Source: CAD feature listing. Evaluate the final solid. Frame: model axes, mm. Face numbers are marked on the shaded views. Coordinates: 2 decimals unless noted, no trailing zeros. Write each loop counter-clockwise with the first axis right and the second up, starting at its lowest first coordinate (ties: lowest second). Pieces come first, ordered by that corner, then holes. Notation, with made-up numbers: M -38,31 L 2,31 A28 cw 2,68 Z; hole C -25.75,38 d8. An arc over 180 degrees is marked long. One line per item, written item: value. Start each with the question number.
Item 1: Pin query (flat end, axial travel): P1, Ø0.7, axis at y = 0.5, z = 8, coming from the +X side. Return the tip coordinate at first contact, or that it passes through.
Item 2: Cut plane B-B, the plane y = 0.75. Output: boundary loops of the cut face in (x, z).
Item 3: Ray query, L1, parallel to X at y = 0.75, z = 4.25; L2, parallel to Y at x = 3.25, z = 4.5; L3, parallel to Y at x = 4.5, z = 7. Return the intervals inside material, ascending. Write a range as from..to.
Item 4: Cut plane A-A, the plane z = 5. Output: boundary loops of the cut face in (x, y).
Item 5: Cut plane C-C, the plane x = 3.5. Output: boundary loops of the cut face in (y, z).
Item 6: Cut plane D-D, the plane x = -3.25. Output: boundary loops of the cut face in (y, z).
Item 7: Mould query, pull axis X, two halves, no side actions, for the marked faces 1, 2 and 3. Classes: released by +X, released by -X, zero draft, split by the parting line, or undercut.
```python
from build123d import *

# Parameters (mm, degrees)
F0_W     = 10
F0_H     = 10
F1_DEPTH = 10
F3_DEPTH = 6


with BuildPart() as f1:
    # F0 (on Top) → F1 (new body)
    with BuildSketch(Plane.XY):
        Rectangle(F0_W, F0_H)
    extrude(amount=F1_DEPTH)

    # F2 (on face) → F3 (cut)
    with BuildSketch(Plane.XY.offset(10)):
        Polygon((-4, 0), (-5, 0), (-5, -1.2), (5, -1.2), (5, 0), (5, 0.9), (4, 0.9), (4, 0), (3, 0), (3, 0.9), (2, 0.9), (2, 0), (1, 0), (1, 0.9), (0, 0.9), (0, 0), (-1, 0), (-1, 0.9), (-2, 0.9), (-2, 0), (-3, 0), (-3, 0.9), (-4, 0.9), align=None)
    extrude(amount=-F3_DEPTH, mode=Mode.SUBTRACT)


solid = f1.part
```
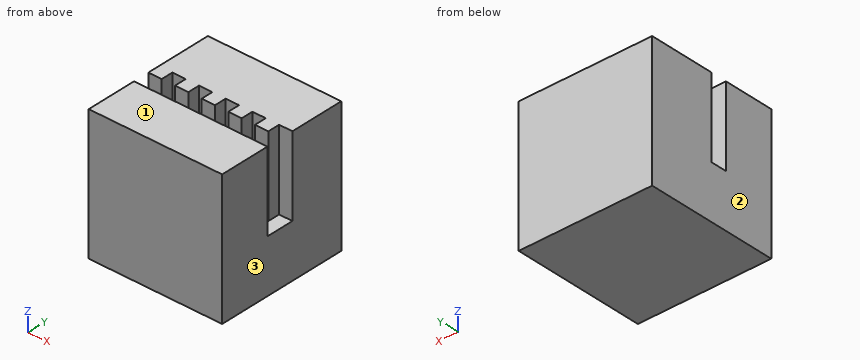
From the geometry:
1. P1: stops at x = 4
2. outline: M -5,0 L 5,0 L 5,4 L 4,4 L 4,10 L 3,10 L 3,4 L 2,4 L 2,10 L 1,10 L 1,4 L 0,4 L 0,10 L -1,10 L -1,4 L -2,4 L -2,10 L -3,10 L -3,4 L -4,4 L -4,10 L -5,10 Z
3. L1: x = -5..-4, -3..-2, -1..0, 1..2, 3..4
3. L2: y = -5..-1.2, 0..5
3. L3: y = -5..-1.2, 0.9..5
4. outline: M -5,-5 L 5,-5 L 5,-1.2 L -5,-1.2 Z; M -5,0 L -4,0 L -4,0.9 L -3,0.9 L -3,0 L -2,0 L -2,0.9 L -1,0.9 L -1,0 L 0,0 L 0,0.9 L 1,0.9 L 1,0 L 2,0 L 2,0.9 L 3,0.9 L 3,0 L 4,0 L 4,0.9 L 5,0.9 L 5,5 L -5,5 Z
5. outline: M -5,0 L 5,0 L 5,10 L 0,10 L 0,4 L -1.2,4 L -1.2,10 L -5,10 Z
6. outline: M -5,0 L 5,0 L 5,10 L 0.9,10 L 0.9,4 L -1.2,4 L -1.2,10 L -5,10 Z
7. face 1: zero draft
7. face 2: released by -X
7. face 3: released by +X
